Could you check a few things on this model? Use its own coordinates, in mm. Face numbers are marked on the shaded views. A direction names the side the tool comes from. Give positions to 0.01 mm unless a question says otherwise; leave off trailing zeros. Loops run counter-clockwise (first coordinate to the right, second up) from the corner with the lowest first, then second, coordinate; pieces in that order, holes last. Notation, with made-up numbers: (-13.75, -27.5) - (-7.75, -27.5) arc R30 ccw to (-7.75, 2.5) - close; hole circle Ø3 at (75.5, -26.75). An arc over 180 degrees is marked (long way). One line per item, written item: value. Start each with the question number.
Q1. If we mould it in two halves opening along X, with no side actions, what happens to the marked faces 1, 2 and 3? For each: released by +X, released by -X, zero draft, split by the parting line, or undercut.
Q2. I want a section at C-C (z = 8.5). Please give me the cut outline in (x, y).
Q3. I want a section at A-A (z = 1.5). Please give me the cut outline in (x, y).
Q4. I want a section at D-D (z = 6.5). Please give me the cut outline in (x, y), then the cut area to 3 significant figures.
Q5. If I drill on line 1 (Y direction, x = 0, z = 17.25); line 2 (Y direction, x = 0.6, z = 19); line 3 (Y direction, x = 0.95, z = 9.5), over which ranges is the centre line in solid material (lowest first)? Write a range as from..to.
Q6. For the marked faces 4 and 5, which set-ups out of +Z, -Z, +X, -X, +Y, -Y let a thin tool reach every point of the face, with its end or its side?
Q7. I want a section at B-B (x = -1.8). Please give me the cut outline in (y, z).
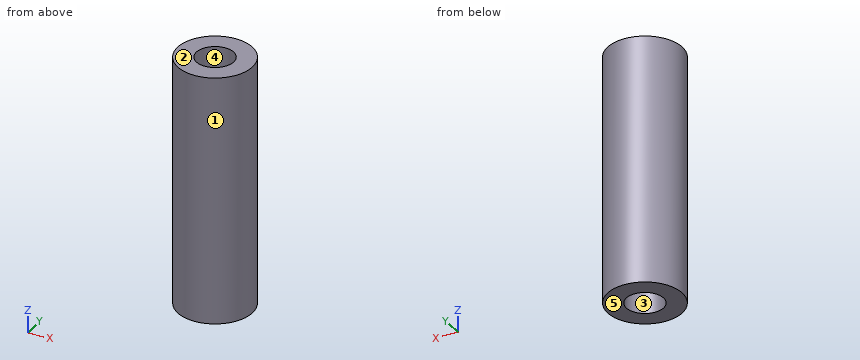
Autodesk Inventor part; units mm, degrees
ref_plane "YZ Plane" through (0, 0, 0) normal (1, 0, 0) x (0, 1, 0)
ref_plane "XZ Plane" through (0, 0, 0) normal (0, 1, 0) x (-1, 0, 0)
ref_plane "XY Plane" through (0, 0, 0) normal (0, 0, 1) x (1, 0, 0)
sketch "スケッチ1" plane through (0, 0, 0) normal (0, 0, 1) x (1, 0, 0)
  circle A0 centre (0, 0) radius 3
  dimension "d0" = 6
extrude "押し出し1" add sketch "スケッチ1" along normal blind 20
hole "穴1" at (0, 0, 0) direction (0, 0, 1) diameter 3 depth 6 tip angle 118
sketch "スケッチ2" plane through (0, 0, 20) normal (0, 0, 1) x (1, 0, 0)
  circle A0 centre (0, 0) radius 3
hole "穴2" at (0, 0, 20) direction (0, 0, -1) diameter 3 depth 6 tip angle 118
properties part number "スペーサ　m3-l20" material "アルミニウム 2014-T4"
Worked answers:
1. face 1: split by the parting line
1. face 2: zero draft
1. face 3: undercut
2. outline: circle Ø6 at (0, 0)
3. outline: circle Ø6 at (0, 0); hole circle Ø3 at (0, 0)
4. outline: circle Ø6 at (0, 0); hole circle Ø1.34 at (0, 0)
4. area: 26.9 mm²
5. line 1: y = -3..-1.5, 1.5..3
5. line 2: y = -2.94..-1.37, 1.37..2.94
5. line 3: y = -2.85..2.85
6. face 4: +Z
6. face 5: -Z, +X, -X, +Y, -Y
7. outline: (-2.4, 0) - (2.4, 0) - (2.4, 20) - (-2.4, 20) - close
